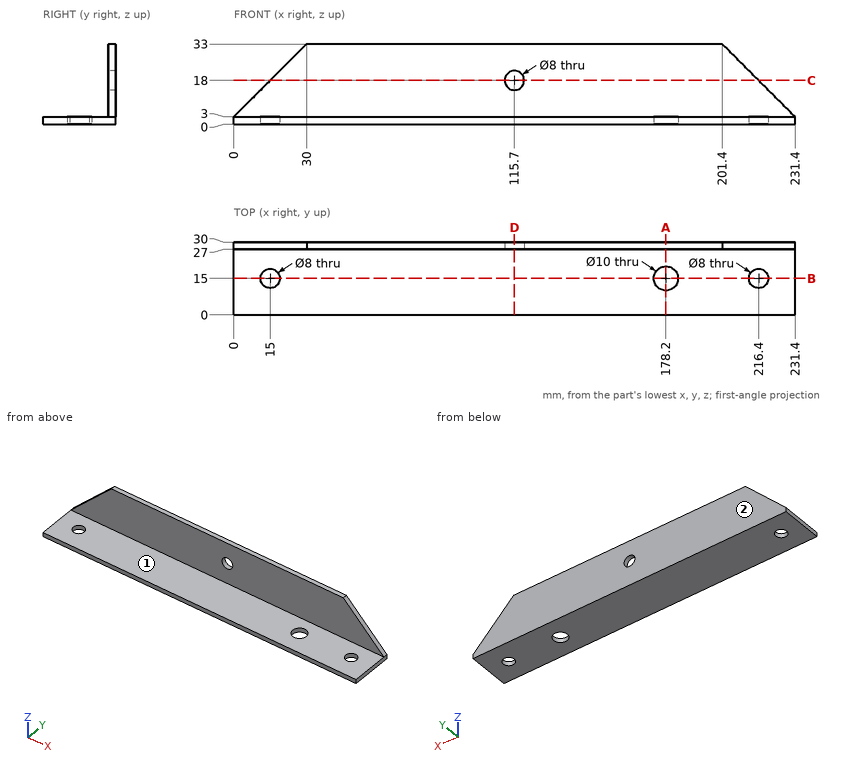
Drawing for the job (mm, zero at the part's lowest x, y, z). A direction names the side the tool comes from. Give positions to 0.01 mm unless a question says otherwise; leave off trailing zeros. Loops run counter-clockwise (first coordinate to the right, second up) from the corner with the lowest first, then second, coordinate; pieces in that order, holes last. Notation, with made-up numbers: (24, 50) - (34, 50) arc R18 cw to (34, 59) - close; hole circle Ø1 at (86, -19). An arc over 180 degrees is marked (long way). Write item = value, one per line. Start each with the question number.
1) Probe probe 1 along Z at (x, y) = (115.7, 27.95); probe 2 along Y at (x, z) = (15, 2.05); probe 3 along Y at (x, z) = (178, 2). List the from-to ranges inside material, lowest first. Write a range as from..to.
2) Tool access for the marked faces 1 and 2: list every direction of +Z, -Z, +X, -X, +Y, -Y with a clear straight run to the whole face (end or side of a thin tool).
3) Band-saw the part on D-D on x = 115.7. Give the cut face in (y, z), plus the area to 3 significant figures.
4) Band-saw the part on A-A on x = 178.2. Give the cut face in (y, z).
5) Band-saw the part on B-B on y = 15. Give the cut face in (x, z).
6) Drop flat-ended pins along their axis: pin 1 Ø4 at (x, z) = (197, 15.5) entering from -Y; pin 2 Ø2 at (x, y) = (206.5, 9) entering from +Z. Give the stop position or say it passes through.
7) Band-saw the part on C-C on z = 18. Give the cut face in (x, y).
Final values:
q1.probe_1 = 0..14, 22..33
q1.probe_2 = 0..11, 19..30
q1.probe_3 = 0..10, 20..30
q2.face_1 = +Z, +X, -X, -Y
q2.face_2 = +Z, -Z, +X, -X, +Y
q3.outline = (0, 0) - (30, 0) - (30, 14) - (27, 14) - (27, 3) - (0, 3) - close; (27, 22) - (30, 22) - (30, 33) - (27, 33) - close
q3.area = 156 mm²
q4.outline = (0, 0) - (10, 0) - (10, 3) - (0, 3) - close; (20, 0) - (30, 0) - (30, 33) - (27, 33) - (27, 3) - (20, 3) - close
q5.outline = (0, 0) - (11, 0) - (11, 3) - (0, 3) - close; (19, 0) - (173.2, 0) - (173.2, 3) - (19, 3) - close; (183.2, 0) - (212.4, 0) - (212.4, 3) - (183.2, 3) - close; (220.4, 0) - (231.4, 0) - (231.4, 3) - (220.4, 3) - close
q6.pin_1 = 27
q6.pin_2 = 3
q7.outline = (15, 27) - (111.7, 27) - (111.7, 30) - (15, 30) - close; (119.7, 27) - (216.4, 27) - (216.4, 30) - (119.7, 30) - close
